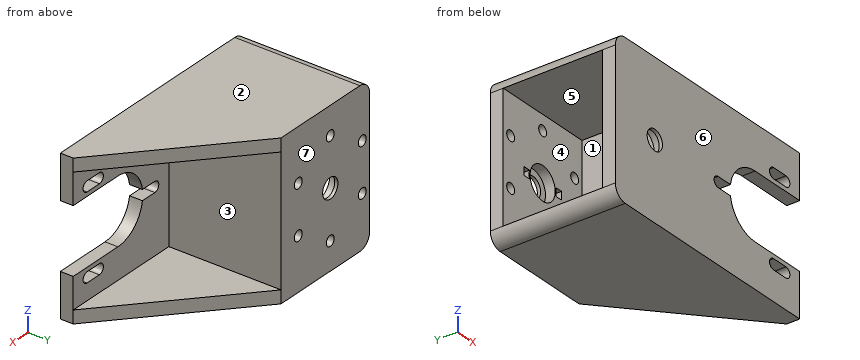
from build123d import *

# Parameters (mm, degrees)
BOSS_EXTRUDE1_DEPTH     = 39.35
CUT_EXTRUDE2_DEPTH      = 33.73
CUT_EXTRUDE2_DEPTH_BACK = 3
SKETCH3_R               = 5.1
CUT_EXTRUDE3_DEPTH      = 33.73
CUT_EXTRUDE4_DEPTH      = 87.647311883
CUT_EXTRUDE4_DEPTH_BACK = 87.647311883
SKETCH3_5_R             = 3.1
SKETCH3_5_R_2           = 10.1
SKETCH3_5_R_3           = 1.6
SKETCH3_5_W             = 20.675
SKETCH3_5_H             = 20.2
SKETCH3_5_W_2           = 5.027537917
SKETCH3_5_H_2           = 3.2
SKETCH3_5_W_3           = 5.03
SKETCH3_6_R             = 1.6
CUT_EXTRUDE5_DEPTH      = 87.647311883
SKETCH4_W               = 77.35
SKETCH4_H               = 38.73
BOSS_EXTRUDE2_DEPTH     = 4
SKETCH5_W               = 77.35
SKETCH5_H               = 38.73
BOSS_EXTRUDE3_DEPTH     = 4
CUT_EXTRUDE6_DEPTH      = 92.909209967
CUT_EXTRUDE6_DEPTH_BACK = 92.909209967
FILLET1_R               = 4


with BuildPart() as part:
    # Sketch1 → Boss-Extrude1 (new body)
    with BuildSketch(Plane.XY):
        Polygon((-68.943174111, 38.106680783), (-32.943174111, 38.106680783), (-32.943174111, 3.376680783), (8.406825889, 3.376680783), (8.406825889, -0.623319217), (-68.943174111, -0.623319217), (-68.943174111, 3.376680783), (-36.943174111, 3.376680783), (-36.943174111, 34.106680783), (-68.943174111, 34.106680783), align=None)
    extrude(amount=BOSS_EXTRUDE1_DEPTH)

    # Sketch3 → Cut-Extrude2 (cut, two sides: drawn at the far end of the back side and taken through both)
    with BuildSketch(Plane(origin=(0, 3.376680783, 0), x_dir=(1, 0, 0), z_dir=(0, 1, 0)).offset(-CUT_EXTRUDE2_DEPTH_BACK)):
        with Locations(Location((-52.943174111, -19.675, 0), (0, 0, 90))):
            Circle(SKETCH3_R)
    extrude(amount=CUT_EXTRUDE2_DEPTH + CUT_EXTRUDE2_DEPTH_BACK, mode=Mode.SUBTRACT)

    # Sketch3<4> → Cut-Extrude3 (cut)
    with BuildSketch(Plane(origin=(0, 3.376680783, 0), x_dir=(1, 0, 0), z_dir=(0, 1, 0))):
        with BuildLine():
            Line((-47.58710279, -20.925), (-45.294644841, -20.925))
            Line((-45.294644841, -20.925), (-45.294644841, -18.425))
            Line((-45.294644841, -18.425), (-47.58710279, -18.425))
            ThreePointArc((-47.58710279, -18.425), (-47.479274758, -19.045870549), (-47.443174111, -19.675))
            ThreePointArc((-47.443174111, -19.675), (-47.479274758, -20.304129451), (-47.58710279, -20.925))
        make_face()
        with BuildLine():
            Line((-60.591703381, -18.425), (-60.591703381, -20.925))
            Line((-60.591703381, -20.925), (-58.299245432, -20.925))
            ThreePointArc((-58.299245432, -20.925), (-58.443174111, -19.675), (-58.299245432, -18.425))
            Line((-58.299245432, -18.425), (-60.591703381, -18.425))
        make_face()
    extrude(amount=CUT_EXTRUDE3_DEPTH, mode=Mode.SUBTRACT)

    # Sketch3<5> → Cut-Extrude4 (cut, two sides: drawn at the far end of the back side and taken through both)
    with BuildSketch(Plane(origin=(0, 3.376680783, 0), x_dir=(1, 0, 0), z_dir=(0, 1, 0)).offset(-CUT_EXTRUDE4_DEPTH_BACK)):
        with Locations(Location((-52.943174111, -19.675, 0), (0, 0, 270))):
            Circle(SKETCH3_5_R)
        with Locations((-12.268174111, -19.675)):
            Circle(SKETCH3_5_R_2)
        with Locations((-4.768174111, -32.665381057)):
            Circle(SKETCH3_5_R_3)
        with Locations((-4.768174111, -6.684618943)):
            Circle(SKETCH3_5_R_3)
        with Locations((-27.268174111, -19.675)):
            Circle(SKETCH3_5_R_3)
        with Locations((0.261825889, -32.665381057)):
            Circle(SKETCH3_5_R_3)
        with Locations((0.261825889, -6.684618943)):
            Circle(SKETCH3_5_R_3)
        with Locations((-1.930674111, -19.675)):
            Rectangle(SKETCH3_5_W, SKETCH3_5_H)
        with Locations((-24.754405152, -19.675)):
            Rectangle(SKETCH3_5_W_2, SKETCH3_5_H_2)
        with Locations((-2.253174111, -32.665381057)):
            Rectangle(SKETCH3_5_W_3, SKETCH3_5_H_2)
        with Locations((-2.253174111, -6.684618943)):
            Rectangle(SKETCH3_5_W_3, SKETCH3_5_H_2)
    extrude(amount=CUT_EXTRUDE4_DEPTH + CUT_EXTRUDE4_DEPTH_BACK, mode=Mode.SUBTRACT)

    # Sketch3<6> → Cut-Extrude5 (cut, through all)
    with BuildSketch(Plane(origin=(0, 3.376680783, 0), x_dir=(1, 0, 0), z_dir=(0, 1, 0))):
        with Locations(Location((-52.943174111, -34.675, 0), (0, 0, 180))):
            Circle(SKETCH3_6_R)
        with Locations(Location((-65.933555168, -27.175, 0), (0, 0, 180))):
            Circle(SKETCH3_6_R)
        with Locations(Location((-65.933555168, -12.175, 0), (0, 0, 180))):
            Circle(SKETCH3_6_R)
        with Locations(Location((-52.943174111, -4.675, 0), (0, 0, 180))):
            Circle(SKETCH3_6_R)
        with Locations(Location((-39.952793054, -12.175, 0), (0, 0, 180))):
            Circle(SKETCH3_6_R)
        with Locations(Location((-39.952793054, -27.175, 0), (0, 0, 180))):
            Circle(SKETCH3_6_R)
    extrude(amount=CUT_EXTRUDE5_DEPTH, mode=Mode.SUBTRACT)

    # Sketch4 → Boss-Extrude2 (add)
    with BuildSketch(Plane.XY.offset(39.35)):
        with Locations((-30.268174111, 18.741680783)):
            Rectangle(SKETCH4_W, SKETCH4_H)
    extrude(amount=BOSS_EXTRUDE2_DEPTH)

    # Sketch5 → Boss-Extrude3 (add)
    with BuildSketch(Plane(origin=(0, 0, 0), x_dir=(-1, 0, 0), z_dir=(0, 0, -1))):
        with Locations((30.268174111, 18.741680783)):
            Rectangle(SKETCH5_W, SKETCH5_H)
    extrude(amount=BOSS_EXTRUDE3_DEPTH)

    # Sketch6 → Cut-Extrude6 (cut, two sides: drawn at the far end of the back side and taken through both)
    with BuildSketch(Plane.XY.offset(43.35).offset(-CUT_EXTRUDE6_DEPTH_BACK)):
        Polygon((-32.943174111, 38.106680783), (5.861825889, 3.376680783), (5.861825889, -0.623319217), (8.406825889, -0.623319217), (8.406825889, 38.106680783), align=None)
    extrude(amount=CUT_EXTRUDE6_DEPTH + CUT_EXTRUDE6_DEPTH_BACK, mode=Mode.SUBTRACT)

    # Fillet1
    fillet1_edges = [part.edges().sort_by_distance(p)[0] for p in [
        (-68.943174111, 18.741680783, 43.35),
        (-68.943174111, 18.741680783, -4),
    ]]
    fillet(fillet1_edges, radius=FILLET1_R - 0.0001)  # a hair under: the kernel refuses the full size


solid = part.part
Check sheet for the modelled part. Datum: model origin and axes. Units: mm. Face numbers are marked on the shaded views. A direction names the side the tool comes from. Round coordinates to 2 decimals unless told otherwise and drop trailing zeros. Loops run counter-clockwise (first coordinate to the right, second up) from the corner with the lowest first, then second, coordinate; pieces in that order, holes last.
1. Sectioned sample at B-B on z = 13. Record the boundary of the cut face in (x, y), and give its area (3 significant figures).
2. Sectioned sample at A-A on x = -19.5. Record the boundary of the cut face in (y, z).
3. Set-up check for the marked faces 1, 2 and 3: record each of +Z, -Z, +X, -X, +Y, -Y from which the full face is reachable in a straight line by a thin tool's end or side.
4. Sectioned sample at C-C on x = -63. Record the boundary of the cut face in (y, z).
5. Gauge pin test, flat ends, axial feed: pin 1 Ø10 at (y, z) = (3.5, 3.5) entering from -X; pin 2 Ø3 at (y, z) = (27.5, 13) entering from -X; pin 3 Ø4 at (y, z) = (8.5, 10.5) entering from +X. Record the tip position at first contact, or that the pin passes through.
6. Scan lines: probe 1 along Z at (x, y) = (-37.5, 30); probe 2 along Y at (x, z) = (-40.5, 8); probe 3 along Y at (x, z) = (-32, 34). Record each from-to range of solid material in increasing order.
7. Mould release check, pull along Y, two halves, no side actions. Record for the marked faces 4, 5, 6 and 7: released by +Y, released by -Y, zero draft, split by the parting line, or undercut.
Recorded:
1. outline: (-68.94, -0.62) - (-19.85, -0.62) - (-19.85, 3.38) - (-32.94, 3.38) - (-32.94, 38.11) - (-38.58, 38.11) - (-38.58, 34.11) - (-36.94, 34.11) - (-36.94, 3.38) - (-68.94, 3.38) - close; (-68.94, 34.11) - (-67.3, 34.11) - (-67.3, 38.11) - (-68.94, 38.11) - close; (-64.56, 34.11) - (-41.32, 34.11) - (-41.32, 38.11) - (-64.56, 38.11) - close
1. area: 441 mm2
2. outline: (-0.62, -4) - (26.08, -4) - (26.08, 0) - (3.38, 0) - (3.38, 12.62) - (-0.62, 12.62) - close; (-0.62, 26.73) - (3.38, 26.73) - (3.38, 39.35) - (26.08, 39.35) - (26.08, 43.35) - (-0.62, 43.35) - close
3. face 1: -X
3. face 2: +Z, +X, -X, +Y, -Y
3. face 3: +X, +Y
4. outline: (-0.62, -4) - (38.11, -4) - (38.11, 43.35) - (-0.62, 43.35) - close; hole (3.38, 0) - (34.11, 0) - (34.11, 39.35) - (3.38, 39.35) - close
5. pin 1: stops at x = -68.94
5. pin 2: stops at x = -36.94
5. pin 3: stops at x = -32.94
6. probe 1: z = -4 to 0, 39.35 to 43.35
6. probe 2: y = -0.62 to 3.38, 34.11 to 38.11
6. probe 3: y = -0.62 to 3.38
7. face 4: undercut
7. face 5: undercut
7. face 6: released by -Y
7. face 7: released by +Y
